Build history of the part. All positions in model axes, mm. A direction names the side the tool comes from. Give positions to 0.01 mm unless a question says otherwise; leave off trailing zeros. Write each loop counter-clockwise with the first axis right and the second up, starting at its lowest first coordinate (ties: lowest second). Pieces come first, ordered by that corner, then holes. Notation, with made-up numbers: M 64.5,36.25 L 112.5,36.25 A16 ccw 112.5,56.25 Z; hole C 11,15 d7. An arc over 180 degrees is marked long. Return JSON: item names as keys, results as strings. Group by question number.
Q1. Wall check: probe 1 along Y at (x, z) = (-16.5, 3.3); probe 2 along X at (y, z) = (-11, 1.9); probe 3 along Z at (x, y) = (-20, 9). Give the ranges that are in metal, low to high.
Q2. Band-saw the part on B-B, the plane z = 2.35. Give the cut face in (x, y).
Q3. Tool access for faces 4 (the flat face through (0, -3, 2)), 5 (the flat face through (-29, -2, 0.75)): list every direction of +Z, -Z, +X, -X, +Y, -Y with a clear straight run to the whole face (end or side of a thin tool).
Q4. Pull direction Y, two halves, no side cores. Call faces 1 (the flat face through (-57.2, -3, 2)), 2 (the flat face through (-29, -54.079, 2)), 3 (the flat face through (-29, 50.171, 2)): +Y half, -Y half, draft (parallel to the pull), parting line (faces both ways), or undercut.
Q5. Flat gauge pin, fed straight in: pin 1 Ø3 at (x, y) = (-13.5, -11.5) entering from +Z. Where does the tip first touch, or does it go through?
Q6. Band-saw the part on A-A, the plane x = -49.5. Give the cut face in (y, z).
Q7. Band-saw the part on C-C, the plane y = -22. Give the cut face in (x, z), then the cut area to 3 significant figures.
from build123d import *

# Parameters (mm, degrees)
F0_W     = 57.2
F0_H     = 105
F1_DEPTH = 4
F2_W     = 55.7
F2_H     = 103.5
F3_DEPTH = 3.25


with BuildPart() as f1:
    # F0 (on Top) → F1 (new body)
    with BuildSketch(Plane.XY):
        with Locations((-28.6, -2.328537)):
            Rectangle(F0_W, F0_H)
    extrude(amount=F1_DEPTH)

    # F2 (on face) → F3 (cut)
    with BuildSketch(Plane.XY.offset(4)):
        with Locations((-28.6, -2.328537)):
            Rectangle(F2_W, F2_H)
    extrude(amount=-F3_DEPTH, mode=Mode.SUBTRACT)


solid = f1.part
From the geometry:
{
 "1": {"probe 1": "y = -54.83 to -54.08, 49.42 to 50.17", "probe 2": "x = -57.2 to -56.45, -0.75 to 0", "probe 3": "z = 0 to 0.75"},
 "2": {"outline": "M -57.2,-54.83 L 0,-54.83 L 0,50.17 L -57.2,50.17 Z; hole M -56.45,-54.08 L -0.75,-54.08 L -0.75,49.42 L -56.45,49.42 Z"},
 "3": {"face 4": "+Z, -Z, +X, +Y, -Y", "face 5": "+Z"},
 "4": {"face 1": "draft", "face 2": "undercut", "face 3": "+Y half"},
 "5": {"pin 1": "stops at z = 0.75"},
 "6": {"outline": "M -54.83,0 L 50.17,0 L 50.17,4 L 49.42,4 L 49.42,0.75 L -54.08,0.75 L -54.08,4 L -54.83,4 Z"},
 "7": {"outline": "M -57.2,0 L 0,0 L 0,4 L -0.75,4 L -0.75,0.75 L -56.45,0.75 L -56.45,4 L -57.2,4 Z", "area": "47.8 mm^2"}
}
